The listing builds one solid part. Answer for the finished solid, in the listing's coordinates (mm). A direction names the side the tool comes from. Coordinates: 2 decimals unless noted, no trailing zeros. Order: outer loops, then holes, each group sorted by start corner. A loop starts at its lowest first (then second) coordinate and runs counter-clockwise, first axis right, second up. Notation, with made-up numbers: (-40, 76.5) -> (-26, 76.5) arc R23 ccw to (-26, 93.5) -> close; hole circle Ø1 at (57.25, 41.5). An arc over 180 degrees is marked (long way). Return JSON: item names as keys, results as strings.
from build123d import *

# Parameters (mm, degrees)
F1_DEPTH = 210
F2_W     = 0.5
F2_H     = 10
F2_H_2   = 68.033398215
F3_DEPTH = 22
F4_R     = 0.5
F6_DEPTH = 5
F7_R     = 3


with BuildPart() as f1:
    # F0 (on Right) → F1 (new body)
    with BuildSketch(Plane.YZ):
        Polygon((30, 0), (30, 30), (20, 30), (1, 11), (1, 9), (-1, 9), (-1, 11), (-20, 30), (-30, 30), (-30, 0), align=None)
    extrude(amount=F1_DEPTH)

    # F2 (on face) → F3 (cut)
    with BuildSketch(Plane.XY.offset(30)):
        with Locations((9.75, 25)):
            Rectangle(F2_W, F2_H)
        with Locations((9.75, -14.0166991075)):
            Rectangle(F2_W, F2_H_2)
    extrude(amount=-F3_DEPTH, mode=Mode.SUBTRACT)

    # F4
    f4_edges = [f1.edges().sort_by_distance(p)[0] for p in [
        (110, -1, 9),
        (110, 1, 9),
        (4.75, -1, 9),
        (4.75, 1, 9),
    ]]
    fillet(f4_edges, radius=F4_R)

    # F5 (on face) → F6 (join)
    with BuildSketch(Plane.YZ.offset(210)):
        with BuildLine():
            Line((20, 30), (-20, 30))
            Line((-20, 30), (-1, 11))
            Line((-1, 11), (-1, 9.5))
            ThreePointArc((-1, 9.5), (-0.8535533906, 9.1464466094), (-0.5, 9))
            Line((-0.5, 9), (0.5, 9))
            ThreePointArc((0.5, 9), (0.8535533906, 9.1464466094), (1, 9.5))
            Line((1, 9.5), (1, 11))
            Line((1, 11), (20, 30))
        make_face()
        with BuildLine():
            Line((-30, 30), (-30, 0))
            Line((-30, 0), (30, 0))
            Line((30, 0), (30, 30))
            Line((30, 30), (20, 30))
            Line((20, 30), (1, 11))
            Line((1, 11), (1, 9.5))
            ThreePointArc((1, 9.5), (0.8535533906, 9.1464466094), (0.5, 9))
            Line((0.5, 9), (-0.5, 9))
            ThreePointArc((-0.5, 9), (-0.8535533906, 9.1464466094), (-1, 9.5))
            Line((-1, 9.5), (-1, 11))
            Line((-1, 11), (-20, 30))
            Line((-20, 30), (-30, 30))
        make_face()
    extrude(amount=F6_DEPTH)

    # F7
    f7_edges = [f1.edges().sort_by_distance(p)[0] for p in [
        (112.5, 30, 30),
        (4.75, 30, 30),
        (112.5, -30, 30),
        (4.75, -30, 30),
        (110, -20, 30),
        (4.75, -20, 30),
        (4.75, 20, 30),
        (110, 20, 30),
        (210, 0, 30),
    ]]
    fillet(f7_edges, radius=F7_R)


solid = f1.part
1. Determine the mould class of faces 4 (the face through (5, -24, 30)), 5 (the face through (109, 10, 20)), 6 (the face through (106, 30, 13)), 7 (the face through (106, -30, 14)) for opening direction Y: pulls with the +Y half, pulls with the -Y half, needs draft (parallel to the pull), parting line crosses it, or undercut.
Answer block:
{"face 4": "needs draft", "face 5": "undercut", "face 6": "pulls with the +Y half", "face 7": "pulls with the -Y half"}
2. The part is cut by section A-A on z = 22. Give the vertices of the cut face in (x, y), and give its area (3 significant figures).
Answer block:
{"outline": "(0, -30) -> (9.5, -30) -> (9.5, -12) -> (0, -12) -> close; (0, 12) -> (9.5, 12) -> (9.5, 30) -> (0, 30) -> close; (10, -30) -> (215, -30) -> (215, 30) -> (10, 30) -> (10, 12) -> (210, 12) -> (210, -12) -> (10, -12) -> close", "area": "7,840 mm2"}
3. The part is cut by section C-C on x = 29.5. Give the vertices of the cut face in (y, z), and give its area (3 significant figures).
Answer block:
{"outline": "(-30, 0) -> (30, 0) -> (30, 27) arc R3 ccw to (27, 30) -> (21.24, 30) arc R3 ccw to (19.12, 29.12) -> (1, 11) -> (1, 9.5) arc R0.5 cw to (0.5, 9) -> (-0.5, 9) arc R0.5 cw to (-1, 9.5) -> (-1, 11) -> (-19.12, 29.12) arc R3 ccw to (-21.24, 30) -> (-27, 30) arc R3 ccw to (-30, 27) -> close", "area": "1,390 mm2"}
4. For faces 1 (the face through (10, -7.1, 16.7)), 2 (the face through (5, -10, 20)), 3 (the face through (112, -22, 30)), determine the directions among +Z, -Z, +X, -X, +Y, -Y from which every point of the face is accessible in a straight line to the end or side of a thin tool.
Answer block:
{"face 1": "+Z, +Y, -Y", "face 2": "+Z, -X", "face 3": "+Z, +X, -X, +Y, -Y"}
5. Consider line 1 (X direction, y = 20.5, z = 18); line 2 (Y direction, x = 23.5, z = 9.5); line 3 (Y direction, x = 179, z = 12). Determine where each line is inside the solid, lowest interval first. Write a range as from..to.
Answer block:
{"line 1": "x = 0..9.5, 10..215", "line 2": "y = -30..-1, 1..30", "line 3": "y = -30..-2, 2..30"}
6. Each of these flat-tipped pins is pushed along its axis until it touches: pin 1 Ø9 at (y, z) = (1.5, 19) entering from -X; pin 2 Ø0.5 at (x, y) = (5, 0) entering from +Z; pin 3 Ø1.5 at (x, y) = (33, -14) entering from +Z. Where does it stop, or does it pass through?
Answer block:
{"pin 1": "stops at x = 210", "pin 2": "stops at z = 9", "pin 3": "stops at z = 24.75"}
7. The part is cut by section D-D on y = -14.5. Give the vertices of the cut face in (x, z).
Answer block:
{"outline": "(0, 0) -> (215, 0) -> (215, 30) -> (213, 30) arc R3 ccw to (210, 27) -> (210, 24.5) -> (10, 24.5) -> (10, 8) -> (9.5, 8) -> (9.5, 24.5) -> (0, 24.5) -> close"}
8. The part is cut by section B-B on y = 7. Give the vertices of the cut face in (x, z).
Answer block:
{"outline": "(0, 0) -> (215, 0) -> (215, 30) -> (213, 30) arc R3 ccw to (210, 27) -> (210, 17) -> (10, 17) -> (10, 8) -> (9.5, 8) -> (9.5, 17) -> (0, 17) -> close"}
